For this review, use the dimensioned drawing (mm, ordinates from the lowest corner) and the shaded views. Coordinates: 2 decimals unless noted, no trailing zeros. Loops run counter-clockwise (first coordinate to the right, second up) from the corner with the lowest first, then second, coordinate; pieces in that order, holes last. Notation, with made-up numbers: (-16.75, -36) -> (9.25, -36) arc R14 cw to (9.25, -30) -> close; hole circle Ø7 at (29.25, 32). An arc over 180 degrees is marked (long way). Answer as a JSON object with one key per item and string values.
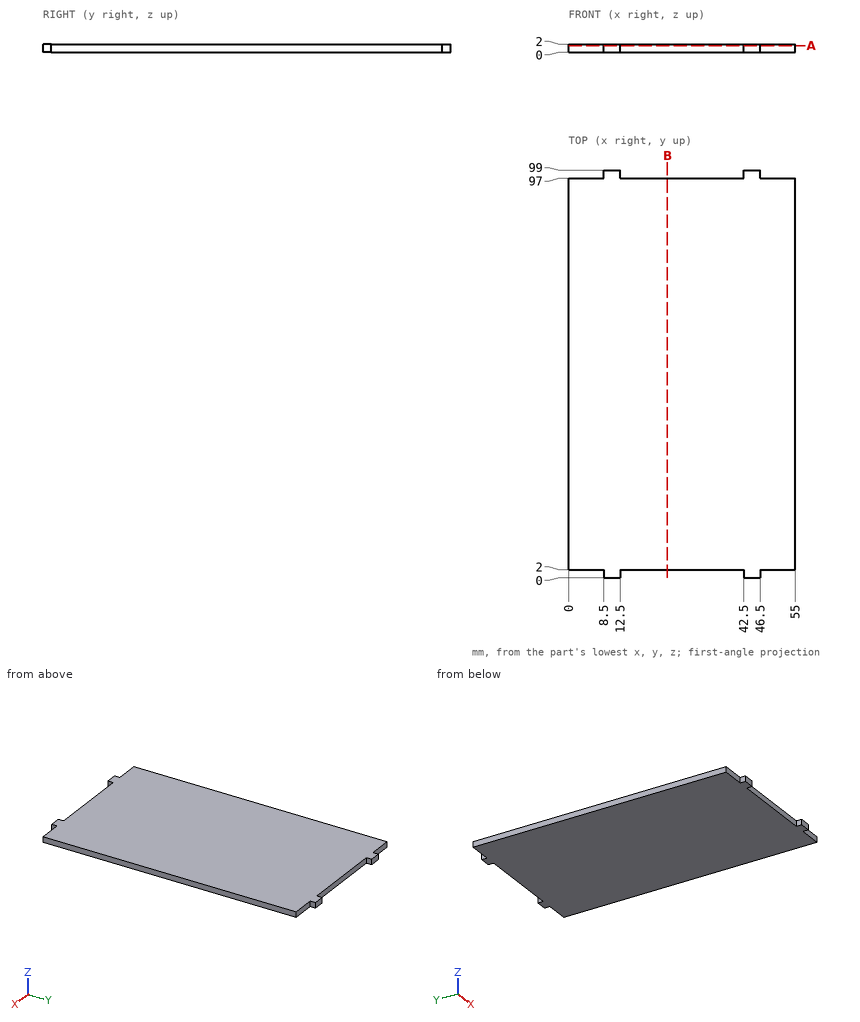
1) Clearance check with flat-ended pins moving along their axes: pin 1 Ø0.6 at (x, z) = (51, 1.5) entering from +Y; pin 2 Ø0.6 at (y, z) = (97.5, 1) entering from +X; pin 3 Ø10 at (x, y) = (8.5, 64.5) entering from -Z. State where each tip first meets the part, or that it passes through.
Completed:
{"pin 1": "y = 97", "pin 2": "x = 46.5", "pin 3": "z = 0"}
2) Add section B-B, the plane x = 24. Give the boundary of the cut face in (y, z).
Completed:
{"outline": "(2, 0) -> (97, 0) -> (97, 2) -> (2, 2) -> close"}
3) Wall thickness on probe 1 along Y at (x, z) = (51, 1): over which ranges is the line inside the solid? List them lowest first.
Completed:
{"probe 1": "2 to 97"}
4) Add section A-A, the plane z = 1.6. Give the boundary of the cut face in (x, y).
Completed:
{"outline": "(0, 2) -> (8.5, 2) -> (8.5, 0) -> (12.5, 0) -> (12.5, 2) -> (42.5, 2) -> (42.5, 0) -> (46.5, 0) -> (46.5, 2) -> (55, 2) -> (55, 97) -> (46.5, 97) -> (46.5, 99) -> (42.5, 99) -> (42.5, 97) -> (12.5, 97) -> (12.5, 99) -> (8.5, 99) -> (8.5, 97) -> (0, 97) -> close"}
